Work out the finished part from the listing and answer in its coordinate system (mm). Coordinates: 2 decimals unless noted, no trailing zeros. Loops run counter-clockwise (first coordinate to the right, second up) from the corner with the lowest first, then second, coordinate; pieces in that order, holes last.
```python
from build123d import *

# Parameters (mm, degrees)
SKETCH1_R           = 25
BOSS_EXTRUDE1_DEPTH = 110
CUT_EXTRUDE1_START  = -100
SKETCH2_R           = 25
SKETCH2_R_2         = 2.5
CUT_EXTRUDE1_DEPTH  = 100
FILLET1_R           = 10


with BuildPart() as part:
    # Sketch1 → Boss-Extrude1 (new body)
    with BuildSketch(Plane(origin=(0, 0, 0), x_dir=(0, 0, -1), z_dir=(1, 0, 0))):
        Circle(SKETCH1_R)
    extrude(amount=BOSS_EXTRUDE1_DEPTH)

    # Sketch2 → Cut-Extrude1 (cut)
    with BuildSketch(Plane(origin=(110, 0, 0), x_dir=(0, 0, -1), z_dir=(1, 0, 0)).offset(CUT_EXTRUDE1_START)):
        Circle(SKETCH2_R)
        Circle(SKETCH2_R_2, mode=Mode.SUBTRACT)
    extrude(amount=CUT_EXTRUDE1_DEPTH, mode=Mode.SUBTRACT)

    # Fillet1
    fillet1_edges = [part.edges().sort_by_distance(p)[0] for p in [
        (0, 0, 25),
    ]]
    fillet(fillet1_edges, radius=FILLET1_R - 0.0001)  # a hair under: the kernel refuses the full size


solid = part.part
```
1. Straight lines are drawn through the part: probe 1 along X at (y, z) = (2.5, 3); probe 2 along Y at (x, z) = (32, 2); probe 3 along Y at (x, z) = (9, 10). For each, find the intervals that lie inside material, in ascending order.
2. Each of these flat-tipped pins is pushed along its axis until it touches: P1, Ø4, axis at y = 3, z = -18, coming from the -X side; P2, Ø6, axis at x = 32.5, y = -2, coming from the -Z side; P3, Ø12, axis at y = 0, z = 14.5, coming from the +X side; P4, Ø12, axis at x = 81.5, z = 10.5, coming from the +Y side. Where does it stop, or does it pass through?
3. Determine the mould class of faces 1 (the cylindrical face through (59.3, -2.44, 0.54)), 2 (the flat face through (110, 0, 0)) for opening direction Y: released by +Y, released by -Y, zero draft, split by the parting line, or undercut.
4. A cutting plane is placed at C-C, the plane x = 11.5. Give the vertices of the cut face in (y, z), then the cut area to 3 significant figures.
Answers below:
1. probe 1: x = 0 to 10
1. probe 2: y = -1.5 to 1.5
1. probe 3: y = -22.86 to 22.86
2. P1: stops at x = 0.08
2. P2: stops at z = -2.5
2. P3: stops at x = 10
2. P4: passes through
3. face 1: split by the parting line
3. face 2: zero draft
4. outline: circle Ø5 at (0, 0)
4. area: 19.6 mm2
